```python
from build123d import *

# Parameters (mm, degrees)
SKETCH1_R           = 1.5
BOSS_EXTRUDE1_DEPTH = 2


with BuildPart() as part:
    # Sketch1 → Boss-Extrude1 (new body)
    with BuildSketch(Plane(origin=(0, 0, 0), x_dir=(1, 0, 0), z_dir=(0, 1, 0))):
        Polygon((-4.5, 3), (0, 5.598076211), (4.5, 3), (10.5, 3), (10.5, -3), (4.5, -3), (0, -5.598076211), (-4.5, -3), (-10.5, -3), (-10.5, 3), align=None)
        with Locations(Location((-7.5, 0, 0), (0, 0, 270))):
            Circle(SKETCH1_R, mode=Mode.SUBTRACT)
        with Locations(Location((7.5, 0, 0), (0, 0, 90))):
            Circle(SKETCH1_R, mode=Mode.SUBTRACT)
    extrude(amount=BOSS_EXTRUDE1_DEPTH)

    # Sketch2 → Revolve1 (revolve)
    with BuildSketch(Plane.XY, mode=Mode.PRIVATE) as revolve1_sk:
        with BuildLine():
            Line((0, -10), (0.5, -10))
            ThreePointArc((0.5, -10), (1.560660172, -9.560660172), (2, -8.5))
            Line((2, -8.5), (2, 2))
            Line((2, 2), (0, 2))
            Line((0, 2), (0, -10))
        make_face()
        Polygon((4, 0), (2, 0), (2, -5.494954839), align=None)
    revolve(revolve1_sk.sketch.rotate(Axis((0, 2, 0), (0, -1, 0)), 180), axis=Axis((0, 2, 0), (0, -1, 0)))


solid = part.part
```
Geometry: final body of the model. Coordinates: model frame, mm. A direction names the side the tool comes from. Coordinates: 2 decimals unless noted, no trailing zeros. Order: outer loops, then holes, each group sorted by start corner. A loop starts at its lowest first (then second) coordinate and runs counter-clockwise, first axis right, second up. Notation, with made-up numbers: (-1.75, 70.25) -> (12.25, 70.25) arc R27 ccw to (12.25, 109.25) -> close; hole circle Ø9 at (45, 15.25). An arc over 180 degrees is marked (long way). Write each question's results on one line, items separated by ' | '. Start each with the question number.
1) First-contact query: pin 1 (2 mm diameter, centred on x = -7.5, y = 1, fed in from -Z); pin 2 (6 mm diameter, centred on x = 0.5, y = -6.5, fed in from -Z); pin 3 (3 mm diameter, centred on y = -1, z = -0.5, fed in from +X); pin 4 (3 mm diameter, centred on y = -2.5, z = -4, fed in from -X). Flat tips, straight axial feed; report the tip coordinate or a pass-through.
2) Mould query, pull axis Z, two halves, no side actions, for faces 1 (the cylindrical face through (9, 1, 0)), 2 (the flat face through (2.219, 0.986, -4.317)), 3 (the flat face through (2.28, 0.99, 4.28)), 4 (the cylindrical face through (-9, 1, 0)). Classes: released by +Z, released by -Z, zero draft, split by the parting line, or undercut.
3) Cut plane A-A, the plane x = 7.5. Output: boundary loops of the cut face in (y, z).
4) Set-up query: faces 5 (the flat face through (8, 1, 3)), 6 (the flat face through (7, 1, -3)), 7 (the flat face through (-7, 1, 3)). Return all of +Z, -Z, +X, -X, +Y, -Y with unobstructed straight access to the full face (end or side cutting, diameter ignored); none if empty.
5) Cut plane C-C, the plane y = -2.25. Output: boundary loops of the cut face in (x, z).
6) Cut plane B-B, the plane z = 0. State how many separate pieces and enclosed holes the cut face has, and give its area (3 significant figures).
7) Cut plane D-D, the plane z = 4.25. Output: boundary loops of the cut face in (x, y), and give its area (3 significant figures).
8) Material intervals for line 1 along X through (y, z) = (1, 0); line 2 along Z through (x, y) = (7.5, 1.65); line 3 along Y through (x, z) = (0, 4.75), sorted ascending.
Checks:
1) pin 1: z = -3 | pin 2: z = -2.71 | pin 3: x = 10.5 | pin 4: x = -2.01
2) face 1: undercut | face 2: released by -Z | face 3: released by +Z | face 4: undercut
3) outline: (0, -3) -> (2, -3) -> (2, -1.5) -> (0, -1.5) -> close; (0, 1.5) -> (2, 1.5) -> (2, 3) -> (0, 3) -> close
4) face 5: +Z, +X, +Y, -Y | face 6: -Z, +X, +Y, -Y | face 7: +Z, -X, +Y, -Y
5) outline: circle Ø6.36 at (0, 0)
6) separate pieces: 3 | enclosed holes: 0 | area: 80.0 mm^2
7) outline: (-2.33, 0) -> (2.33, 0) -> (2.33, 2) -> (-2.33, 2) -> close | area: 9.34 mm^2
8) line 1: -10.5 to -9, -6 to 6, 9 to 10.5 | line 2: -3 to -1.5, 1.5 to 3 | line 3: 0 to 2
